Work out the finished part from the listing and answer in its coordinate system (mm). A direction names the side the tool comes from. Coordinates: 2 decimals unless noted, no trailing zeros. Order: outer loops, then holes, each group sorted by start corner. A loop starts at its lowest first (then second) coordinate and runs counter-clockwise, first axis right, second up. Notation, with made-up numbers: (26, 85.5) -> (46, 85.5) arc R9 cw to (46, 102.5) -> close; hole circle Ø6 at (-20, -18). An arc over 180 degrees is marked (long way). Use one line per item in the form item = value.
Autodesk Inventor part; units mm, degrees
ref_plane "YZ Plane" through (0, 0, 0) normal (1, 0, 0) x (0, 1, 0)
ref_plane "XZ Plane" through (0, 0, 0) normal (0, 1, 0) x (-1, 0, 0)
ref_plane "XY Plane" through (0, 0, 0) normal (0, 0, 1) x (1, 0, 0)
sketch "Sketch1" plane through (0, 0, 0) normal (0, 0, 1) x (1, 0, 0)
  circle A0 centre (0, 0) radius 16
  dimension "d0" = 32
extrude "Extrusion1" add sketch "Sketch1" against normal blind 9
sketch "Sketch2" plane through (0, 0, 0) normal (0, 0, 1) x (1, 0, 0)
  circle A0 centre (0, 0) radius 16
  circle A1 centre (0, 0) radius 16
  circle A2 centre (0, 0) radius 12
  dimension "d3" = 32
  dimension "d4" = 24
extrude "Extrusion2" cut sketch "Sketch2" against normal blind 1.5
sketch "Sketch3" plane through (0, 0, 0) normal (0, 0, 1) x (1, 0, 0)
  circle A0 centre (0, 0) radius 12
  arc A1 (-1.118, 1) -> (1.118, 1) centre (0, 0) ccw
  line L0 (0, 0) -> (0, 1)
  line L1 (0, 1) -> (-1.118, 1)
  line L2 (0, 1) -> (1.118, 1)
  arc A2 (1.118, 1) -> (-1.118, 1) centre (0, 0) ccw
  dimension "d7" = 3
  dimension "d8" = 1
extrude "Extrusion3" cut sketch "Sketch3" against normal blind 8 contours L1 L2 A1
properties part number "Wheel"
(1) Each of these flat-tipped pins is pushed along its axis until it touches: P1, Ø1.5, axis at x = -5.5, z = -5.5, coming from the -Y side; P2, Ø4, axis at x = -7.5, z = -6.5, coming from the -Y side (3 decimals); P3, Ø2, axis at x = 7.5, z = -7, coming from the -Y side. Where does it stop, or does it pass through?
Data:
P1 = -15.28
P2 = -15.025
P3 = -14.62
(2) Section B-B on y = 0 is taken. Write down the section's boundary in (x, z).
Data:
outline = (-16, -9) -> (16, -9) -> (16, -1.5) -> (12, -1.5) -> (12, 0) -> (1.5, 0) -> (1.5, -8) -> (-1.5, -8) -> (-1.5, 0) -> (-12, 0) -> (-12, -1.5) -> (-16, -1.5) -> close
(3) Which of the six approach directions +Z, -Z, +X, -X, +Y, -Y give full straight-line access (tool end or side, diameter ignored) to faces 1 (the flat face through (0, 1, -4)), 2 (the flat face through (2, 0, 0))?
Data:
face_1 = +Z
face_2 = +Z, +X, -X, +Y, -Y
(4) Section C-C on x = 0 is taken. Write down the section's boundary in (y, z), plus the area to 3 significant figures.
Data:
outline = (-16, -9) -> (16, -9) -> (16, -1.5) -> (12, -1.5) -> (12, 0) -> (1, 0) -> (1, -8) -> (-1.5, -8) -> (-1.5, 0) -> (-12, 0) -> (-12, -1.5) -> (-16, -1.5) -> close
area = 256 mm²
(5) Section D-D on z = -2.75 is taken. Write down the section's boundary in (x, y), plus the area to 3 significant figures.
Data:
outline = circle Ø32 at (0, 0); hole (-1.12, 1) arc R1.5 ccw (long way) to (1.12, 1) -> close
area = 798 mm²
(6) The mould has two halves that part along X. Classify faces 3 (the flat face through (0, 0, -9)), 4 (the flat face through (0, 0, -8)), 5 (the cylindrical face through (-3.47, -15.62, -5.2)): released by +X, released by -X, zero draft, split by the parting line, or undercut.
Data:
face_3 = zero draft
face_4 = undercut
face_5 = split by the parting line
(7) Section A-A on z = -1 is taken. Write down the section's boundary in (x, y).
Data:
outline = circle Ø24 at (0, 0); hole (-1.12, 1) arc R1.5 ccw (long way) to (1.12, 1) -> close
(8) Straight lines are drawn through the part: line 1 along Y through (x, z) = (-1, -4.25); line 2 along Z through (x, y) = (11.5, 6); line 3 along Y through (x, z) = (14.5, -8.25). For each, find the intervals that lie inside material, in ascending order.
Data:
line_1 = -15.97 to -1.12, 1 to 15.97
line_2 = -9 to -1.5
line_3 = -6.76 to 6.76
